from build123d import *

# Parameters (mm, degrees)
SKETCH1_W                = 54
SKETCH1_H                = 20
BOSS_EXTRUDE1_DEPTH      = 5
SKETCH2_W                = 54
SKETCH2_H                = 5
BOSS_EXTRUDE2_DEPTH      = 10.8
M3_CLEARANCE_HOLE1_D     = 3.4
M3_CLEARANCE_HOLE1_DEPTH = 28.71
M3_CLEARANCE_HOLE1_TIP   = 1.021463052
M3_CLEARANCE_HOLE2_D     = 3.4
FILLET1_R                = 5
SKETCH11_R               = 2.35
CUT_EXTRUDE4_DEPTH       = 7.8
SKETCH9_R                = 2.35
CUT_EXTRUDE5_DEPTH       = 7.8


with BuildPart() as part:
    # Sketch1 → Boss-Extrude1 (new body)
    with BuildSketch(Plane(origin=(0, 0, 0), x_dir=(1, 0, 0), z_dir=(0, 1, 0))):
        Rectangle(SKETCH1_W, SKETCH1_H)
    extrude(amount=BOSS_EXTRUDE1_DEPTH)

    # Sketch2 → Boss-Extrude2 (add)
    with BuildSketch(Plane(origin=(0, 5, 0), x_dir=(1, 0, 0), z_dir=(0, 1, 0))):
        with Locations((0, 7.5)):
            Rectangle(SKETCH2_W, SKETCH2_H)
    extrude(amount=BOSS_EXTRUDE2_DEPTH)

    # M3 Clearance Hole1
    with Locations(Plane.XY.offset(-5)):
        with Locations((-13.75, 12.6), (13.75, 12.6)):
            Hole(M3_CLEARANCE_HOLE1_D / 2, depth=M3_CLEARANCE_HOLE1_DEPTH)
            with Locations((0, 0, -(M3_CLEARANCE_HOLE1_DEPTH + M3_CLEARANCE_HOLE1_TIP / 2))):  # 118° drill point
                Cone(0, M3_CLEARANCE_HOLE1_D / 2, M3_CLEARANCE_HOLE1_TIP, mode=Mode.SUBTRACT)

    # M3 Clearance Hole2 (through all)
    with Locations(Plane(origin=(0, 5, 0), x_dir=(1, 0, 0), z_dir=(0, 1, 0))):
        with Locations((15, -2), (-15, -2)):
            Hole(M3_CLEARANCE_HOLE2_D / 2)

    # Fillet1
    fillet1_edges = [part.edges().sort_by_distance(p)[0] for p in [
        (27, 2.5, 10),
        (-27, 2.5, 10),
        (27, 15.8, -7.5),
        (-27, 15.8, -7.5),
    ]]
    fillet(fillet1_edges, radius=FILLET1_R)

    # Sketch11 → Cut-Extrude4 (cut)
    with BuildSketch(Plane(origin=(0, 0, -10), x_dir=(-1, 0, 0), z_dir=(0, 0, -1))):
        with Locations((-13.75, 11.95)):
            Circle(SKETCH11_R)
    extrude(amount=-CUT_EXTRUDE4_DEPTH, mode=Mode.SUBTRACT)

    # Sketch9 → Cut-Extrude5 (cut)
    with BuildSketch(Plane(origin=(0, 0, -10), x_dir=(-1, 0, 0), z_dir=(0, 0, -1))):
        with Locations((13.75, 11.95)):
            Circle(SKETCH9_R)
    extrude(amount=-CUT_EXTRUDE5_DEPTH, mode=Mode.SUBTRACT)


solid = part.part
The listing builds one solid part. Answer for the finished solid, in the listing's coordinates (mm). A direction names the side the tool comes from. Coordinates: 2 decimals unless noted, no trailing zeros. Write each loop counter-clockwise with the first axis right and the second up, starting at its lowest first coordinate (ties: lowest second). Pieces come first, ordered by that corner, then holes. Notation, with made-up numbers: (44, 67) - (77, 67) arc R18 cw to (77, 78) - close; hole circle Ø11 at (-2.75, -9.75). An arc over 180 degrees is marked (long way). Put each result on its own line as item: value.
1. A tool of negligible diameter and unlimited length cuts with its end or side. For faces 4 (the face through (0, 5, 2)), 5 (the face through (0, 8, -10)), from which of +Z, -Z, +X, -X, +Y, -Y can it reach the whole face along a straight path? Write none if from no direction.
Answer sheet:
face 4: +Z, +X, -X, +Y
face 5: -Z, +X, -X, +Y, -Y
2. Find the intervals of material crossed by line 1 along Y through (x, z) = (13.75, -8.3); line 2 along Z through (x, y) = (15, 2.6); line 3 along X through (y, z) = (4, 2.25), in increasing order. Write a range as from..to.
Answer sheet:
line 1: y = 0..9.6, 14.3..15.8
line 2: z = -10..0.3, 3.7..10
line 3: x = -27..-16.68, -13.32..13.32, 16.68..27
3. The part is cut by section D-D on x = -9. Give the vertices of the cut face in (y, z).
Answer sheet:
outline: (0, -10) - (15.8, -10) - (15.8, -5) - (5, -5) - (5, 10) - (0, 10) - close
4. The part is cut by section C-C on y = 11.95. Give the vertices of the cut face in (x, z).
Answer sheet:
outline: (-26.87, -10) - (-16.1, -10) - (-16.1, -5) - (-26.87, -5) - close; (-11.4, -10) - (11.4, -10) - (11.4, -5) - (-11.4, -5) - close; (16.1, -10) - (26.87, -10) - (26.87, -5) - (16.1, -5) - close
5. The part is cut by section B-B on x = 15. Give the vertices of the cut face in (y, z), plus the area to 3 significant figures.
Answer sheet:
outline: (0, -10) - (9.96, -10) - (9.96, -5) - (5, -5) - (5, 0.3) - (0, 0.3) - close; (0, 3.7) - (5, 3.7) - (5, 10) - (0, 10) - close; (13.94, -10) - (15.8, -10) - (15.8, -5) - (13.94, -5) - close
area: 117 mm^2
6. Flat-ended cylindrical pins translate along their axes: pin 1 Ø5.5 at (x, y) = (13.75, 11.95) entering from +Z; pin 2 Ø7.5 at (x, z) = (-7, 5) entering from +Y; pin 3 Ø3 at (x, z) = (11.5, 3) entering from -Y; pin 4 Ø4 at (x, y) = (-13.75, 11.95) entering from +Z. Find the tip coordinate at first contact, or state that the pin passes through.
Answer sheet:
pin 1: stops at z = -5
pin 2: stops at y = 5
pin 3: stops at y = 0
pin 4: passes through
7. The part is cut by section A-A on z = 2. Give the vertices of the cut face in (x, y), plus the area to 3 significant figures.
Answer sheet:
outline: (-27, 0) - (-16.7, 0) - (-16.7, 5) - (-27, 5) - close; (-13.3, 0) - (13.3, 0) - (13.3, 5) - (-13.3, 5) - close; (16.7, 0) - (27, 0) - (27, 5) - (16.7, 5) - close
area: 236 mm^2
8. Determine the mould class of faces 1 (the face through (-16.57, 2.47, 2.65)), 2 (the face through (0, 10, -5)), 3 (the face through (0, 15.8, -8)) for opening direction Z: pulls with the +Z half, pulls with the -Z half, needs draft (parallel to the pull), parting line crosses it, or undercut.
Answer sheet:
face 1: undercut
face 2: pulls with the +Z half
face 3: needs draft
